Design review of the part built by this model. Coordinates are the model's own, in mm. A direction names the side the tool comes from. Round coordinates to 2 decimals unless told otherwise and drop trailing zeros. Write each loop counter-clockwise with the first axis right and the second up, starting at its lowest first coordinate (ties: lowest second). Pieces come first, ordered by that corner, then holes. Notation, with made-up numbers: (59.25, 9.5) - (111.25, 9.5) arc R10 ccw to (111.25, 22.5) - close; hole circle Ø9 at (43, -8). An arc over 180 degrees is marked (long way). Use one line per item in the form item = value.
Autodesk Inventor part; units mm, degrees
ref_plane "Work Plane1" through (0, 6, 0) normal (0, 1, 0) x (-1, 0, 0)
ref_plane "YZ Plane" through (0, 0, 0) normal (1, 0, 0) x (0, 1, 0)
ref_plane "XZ Plane" through (0, 0, 0) normal (0, 1, 0) x (-1, 0, 0)
sketch "Sketch1" plane through (0, 0, 0) normal (0, 0, 1) x (1, 0, 0)
  circle A0 centre (0, 0) radius 4
  circle A1 centre (0, 0) radius 6
  dimension "d0" = 8
  dimension "d1" = 2
extrude "Extrusion1" add sketch "Sketch1" along normal blind 10
sketch "Sketch2" plane through (0, 0, 10) normal (0, 0, 1) x (1, 0, 0)
  circle A0 centre (0, 0) radius 4
  dimension "d4" = 8
extrude "Extrusion2" add sketch "Sketch2" along normal mid plane 6
move faces "Move1" translate (0, 0, 2.5) faces at (0.7574, 1.0973, 13)
sketch "Sketch3" plane through (0, 0, 0) normal (0, 0, -1) x (-1, 0, 0)
  line L0 (0, 0) -> (0, 6)
  circle A0 centre (0, 0) radius 6
ref_plane "Work Plane1" through (0, 6, 0) normal (0, 1, 0) x (-1, 0, 0)
sketch "Sketch4" plane through (0, 6, 0) normal (0, 1, 0) x (-1, 0, 0)
  circle A0 centre (0, 4.3) radius 1.5
  point P0 (0, 0)
  dimension "d10" = 3
  dimension "d11" = 4.3
extrude "Extrusion3" cut sketch "Sketch4" against normal through all
properties part number "shaft_extension"
Q1. We need section B-B on y = 0. Write out the cut boundary in (x, z), then the cut area to 3 significant figures.
Calculated:
outline = (-6, 0) - (-4, 0) - (-4, 7) - (4, 7) - (4, 0) - (6, 0) - (6, 10) - (4, 10) - (4, 15.5) - (-4, 15.5) - (-4, 10) - (-6, 10) - close
area = 108 mm2
Q2. We need section D-D on y = 5.25. Write out the cut boundary in (x, z), then the cut area to 3 significant figures.
Calculated:
outline = (-2.9, 0) - (2.9, 0) - (2.9, 10) - (-2.9, 10) - close; hole circle Ø3 at (0, 4.3)
area = 51.0 mm2
Q3. Draft analysis for pull direction Z (two halves, no side actions). For faces 1 (the cylindrical face through (1.11, 4.87, 5.31)), 2 (the flat face through (-1.42, -3.92, 10)), 3 (the flat face through (-1.42, -3.92, 0)), 4 (the cylindrical face through (-0.867, 3.905, 12.712)), state which applies: released by +Z, released by -Z, zero draft, split by the parting line, or undercut.
Calculated:
face_1 = undercut
face_2 = released by +Z
face_3 = released by -Z
face_4 = zero draft
Q4. We need section C-C on z = 4.3. Write out the cut boundary in (x, y).
Calculated:
outline = (-1.5, -5.81) - (-1.5, -3.71) arc R4 cw to (-1.5, 3.71) - (-1.5, 5.81) arc R6 ccw to start; (1.5, -5.81) arc R6 ccw to (1.5, 5.81) - (1.5, 3.71) arc R4 cw to (1.5, -3.71) - close
Q5. To check wall thickness, follow line 1 along Z through (x, y) = (0, 5.45); line 2 along X through (y, z) = (0, 4.25); line 3 along Z through (x, y) = (-4, -0.75). State the ranges of each line that lie inside material, in increasing order. Write a range as from..to.
Calculated:
line_1 = 0..2.8, 5.8..10
line_2 = -6..-4, 4..6
line_3 = 0..10
Q6. Machinability: for faces 5 (the flat face through (0, 0, 15.5)), 6 (the cylindrical face through (3.695, 1.532, 3.451)), which of the approach directions +Z, -Z, +X, -X, +Y, -Y give a long, thin tool a straight path to every point of the face, cutting with its end or side? Answer none if there is none.
Calculated:
face_5 = +Z, +X, -X, +Y, -Y
face_6 = -Z
Q7. We need section A-A on x = 0. Write out the cut boundary in (y, z).
Calculated:
outline = (-6, 0) - (-4, 0) - (-4, 2.8) - (-6, 2.8) - close; (-6, 5.8) - (-4, 5.8) - (-4, 7) - (4, 7) - (4, 5.8) - (6, 5.8) - (6, 10) - (4, 10) - (4, 15.5) - (-4, 15.5) - (-4, 10) - (-6, 10) - close; (4, 0) - (6, 0) - (6, 2.8) - (4, 2.8) - close
Q8. For P1, Ø3, axis at x = 3, z = 3, coming from the -Y side; P2, Ø3, axis at y = 4, z = 3, coming from the +X side, all flat-tipped, find the tip position at first contact; note any pin that passes through.
Calculated:
P1 = -5.81
P2 = 5.45
